Answer from the drawing. Dimensions are ordinates in mm from the lowest x, y and z of the part. Round coordinates to 2 decimals unless told otherwise and drop trailing zeros. Write each loop counter-clockwise with the first axis right and the second up, starting at its lowest first coordinate (ties: lowest second). Pieces come first, ordered by that corner, then holes. Notation, with made-up numbers: (-14, 61.5) - (35, 61.5) arc R22 cw to (35, 80.5) - close; hole circle Ø6 at (69, -32). An arc over 180 degrees is marked (long way). Answer in a Markdown table with one row per item.
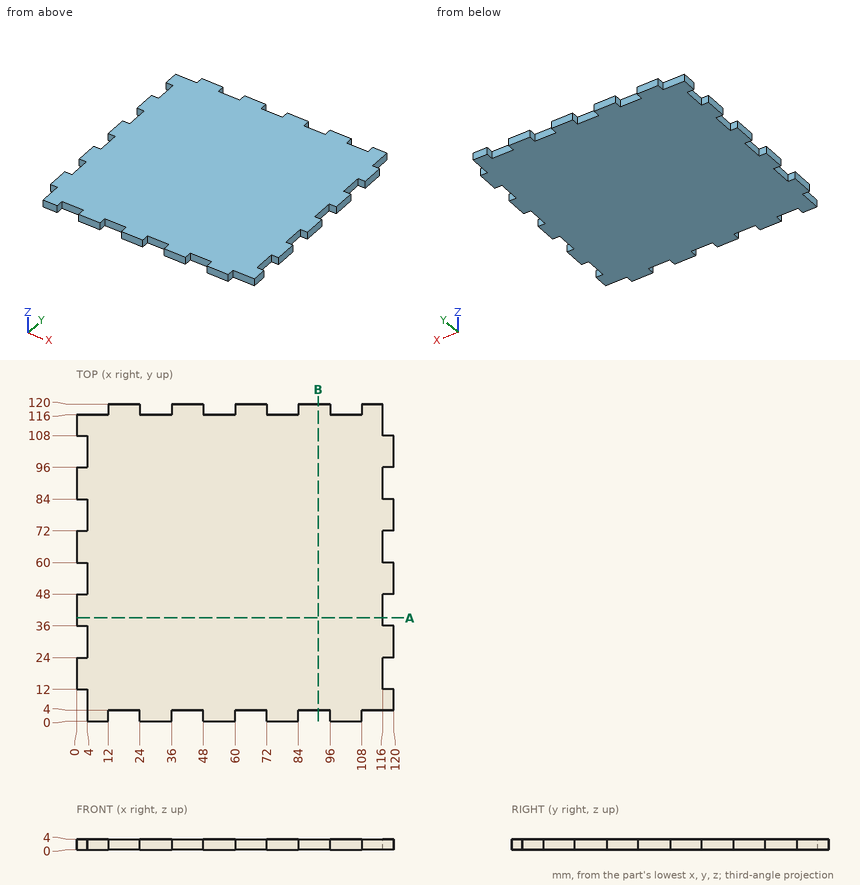
(1) Section A-A (y = 39) is taken. Give the vertices of the cut face in (x, z).
Checked values:
| item | result |
|---|---|
| outline | (0, 0) - (116, 0) - (116, 4) - (0, 4) - close |
(2) Find the intervals of material crossed by line 1 (Y direction, x = 109.5, z = 1.75); line 2 (Y direction, x = 104, z = 1.6), in increasing order.
Checked values:
| item | result |
|---|---|
| line 1 | y = 4 to 120 |
| line 2 | y = 0 to 116 |
(3) Section B-B (x = 91.5) is taken. Give the vertices of the cut face in (y, z).
Checked values:
| item | result |
|---|---|
| outline | (4, 0) - (120, 0) - (120, 4) - (4, 4) - close |
(4) Flat-ended cylindrical pins translate along their axes: pin 1 (1.2 mm diameter, centred on x = 3, z = 1.5, fed in from -Y); pin 2 (1.2 mm diameter, centred on y = 118.5, z = 2, fed in from +X); pin 3 (1.2 mm diameter, centred on y = 29.5, z = 2, fed in from -X). Find the tip coordinate at first contact, or state that the pin passes through.
Checked values:
| item | result |
|---|---|
| pin 1 | stops at y = 12 |
| pin 2 | stops at x = 116 |
| pin 3 | stops at x = 4 |
